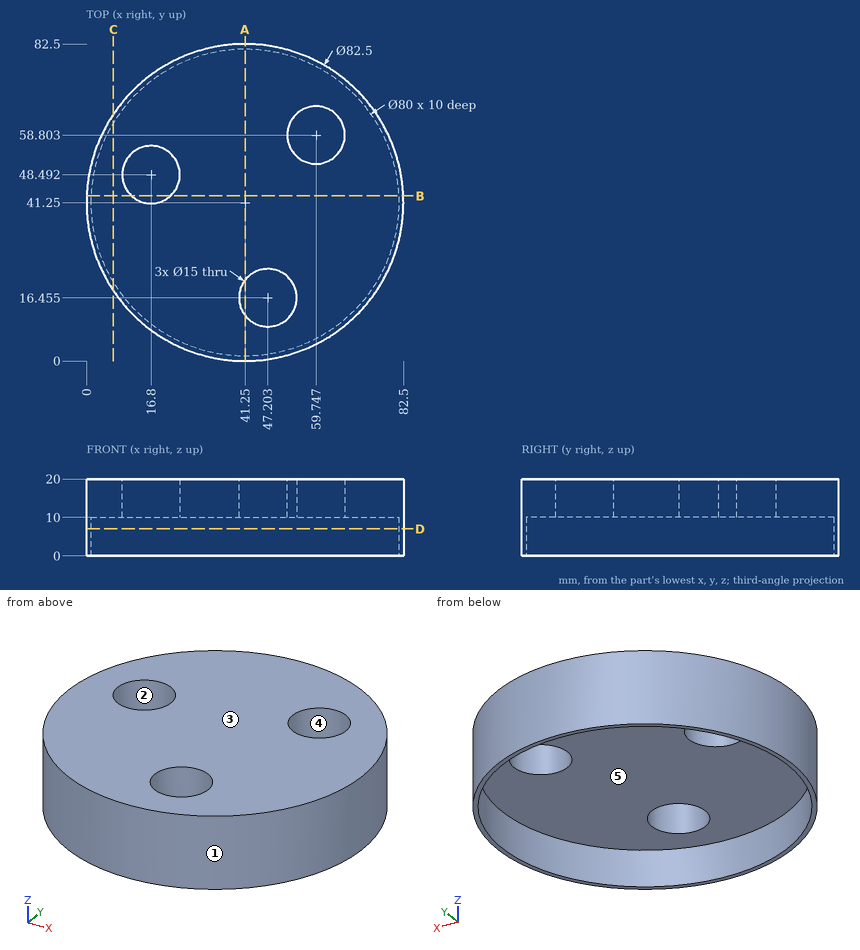
Geometry: see drawing. Coordinates: mm, zero at the bounding-box minimum. A direction names the side the tool comes from. Round coordinates to 2 decimals unless told otherwise and drop trailing zeros. Order: outer loops, then holes, each group sorted by start corner. A loop starts at its lowest first (then second) coordinate and runs counter-clockwise, first axis right, second up. Notation, with made-up numbers: (64.5, 64.5) -> (107.5, 64.5) arc R29 ccw to (107.5, 90.5) -> close; hole circle Ø2 at (-33.75, 43.5). An arc over 180 degrees is marked (long way). Use CSV: the item, a comma, the result in double quotes.
(1) Access query for the marked faces 4 and 5. Directions: +Z, -Z, +X, -X, +Y, -Y. A direction counts if a zero-diameter tool reaches every point of the face in a straight line with its end or side. Return the directions, or none.
Report:
face 4,"+Z, -Z"
face 5,"-Z"
(2) Section C-C on x = 7. Return the cut outline in (y, z), and give its area (3 significant figures).
Report:
outline,"(18.26, 0) -> (20.59, 0) -> (20.59, 10) -> (61.91, 10) -> (61.91, 0) -> (64.24, 0) -> (64.24, 20) -> (18.26, 20) -> close"
area,"506 mm^2"
(3) Section D-D on z = 7. Return the cut outline in (x, y), and give its area (3 significant figures).
Report:
outline,"circle Ø82.5 at (41.25, 41.25); hole circle Ø80 at (41.25, 41.25)"
area,"319 mm^2"
(4) Pull-direction query (Y, two-part tool) for the marked faces 1, 2 and 3; classes: +Y half, -Y half, draft (parallel to the pull), parting line (faces both ways), or undercut.
Report:
face 1,"parting line"
face 2,"undercut"
face 3,"draft"
(5) First-contact query: pin 1 Ø6 at (y, z) = (56, 7) entering from -X; pin 2 Ø24 at (x, y) = (47.2, 16.45) entering from -Z; pin 3 Ø6 at (y, z) = (24, 15.5) entering from -X; pin 4 Ø9 at (x, y) = (16.8, 48.49) entering from -Z. Flat tips, straight axial feed; report the tip coordinate or a pass-through.
Report:
pin 1,"x = 1.71"
pin 2,"z = 10"
pin 3,"x = 2.54"
pin 4,"through"
(6) Section B-B on y = 43. Return the cut outline in (x, z), and give its area (3 significant figures).
Report:
outline,"(0.04, 0) -> (1.29, 0) -> (1.29, 10) -> (11.69, 10) -> (11.69, 20) -> (0.04, 20) -> close; (21.91, 10) -> (81.21, 10) -> (81.21, 0) -> (82.46, 0) -> (82.46, 20) -> (21.91, 20) -> close"
area,"747 mm^2"
(7) Ray query, L1, parallel to Y at x = 41.25, z = 6.25; L2, parallel to X at y = 42.5, z = 8.75; L3, parallel to Z at x = 7, y = 37.5. Return the intervals inside material, ascending.
Report:
L1,"0 to 1.25, 81.25 to 82.5"
L2,"0.02 to 1.27, 81.23 to 82.48"
L3,"10 to 20"
(8) Section A-A on x = 41.25. Return the cut outline in (y, z).
Report:
outline,"(0, 0) -> (1.25, 0) -> (1.25, 10) -> (11.89, 10) -> (11.89, 20) -> (0, 20) -> close; (21.02, 10) -> (81.25, 10) -> (81.25, 0) -> (82.5, 0) -> (82.5, 20) -> (21.02, 20) -> close"
